```python
from build123d import *

# Parameters (mm, degrees)
F0_R     = 5
F1_DEPTH = 6.35
F0_R_2   = 11.43
F2_DEPTH = 3.175
F3_R     = 1.27


with BuildPart() as f1:
    # F0 (on Top) → F1 (new body)
    with BuildSketch(Plane.XY):
        Circle(F0_R)
    extrude(amount=F1_DEPTH)

    # F0 (on Top) → F2 (join)
    with BuildSketch(Plane.XY):
        Circle(F0_R_2)
        Circle(F0_R, mode=Mode.SUBTRACT)
    extrude(amount=F2_DEPTH)

    # F3
    f3_edges = [f1.edges().sort_by_distance(p)[0] for p in [
        (-11.43, 0, 0),
    ]]
    fillet(f3_edges, radius=F3_R)


solid = f1.part
```
Geometry: final body of the model. Coordinates: model frame, mm. A direction names the side the tool comes from. Round coordinates to 2 decimals unless told otherwise and drop trailing zeros. Write each loop counter-clockwise with the first axis right and the second up, starting at its lowest first coordinate (ties: lowest second). Pieces come first, ordered by that corner, then holes. Notation, with made-up numbers: (16, 17.25) -> (71, 17.25) arc R5 cw to (71, 21.25) -> close; hole circle Ø4 at (2.25, 71). An arc over 180 degrees is marked (long way). Return JSON: item names as keys, results as strings.
Q1. First-contact query: pin 1 Ø1.5 at (y, z) = (3.5, 2.5) entering from +X; pin 2 Ø1 at (x, z) = (3, 2.5) entering from +Y; pin 3 Ø1.5 at (x, y) = (5.5, -3.5) entering from +Z (3 decimals). Flat tips, straight axial feed; report the tip coordinate or a pass-through.
From the geometry:
{"pin 1": "x = 11.09", "pin 2": "y = 11.15", "pin 3": "z = 3.175"}
Q2. Section C-C on z = 4.25. Return the cut outline in (x, y).
From the geometry:
{"outline": "circle Ø10 at (0, 0)"}
Q3. Section A-A on y = 0. Return the cut outline in (x, z) (3 decimals).
From the geometry:
{"outline": "(-11.43, 1.27) arc R1.27 ccw to (-10.16, 0) -> (10.16, 0) arc R1.27 ccw to (11.43, 1.27) -> (11.43, 3.175) -> (5, 3.175) -> (5, 6.35) -> (-5, 6.35) -> (-5, 3.175) -> (-11.43, 3.175) -> close"}
Q4. Ray query, line 1 (Z direction, x = -9.25, y = -2.5) (3 decimals); line 2 (Y direction, x = -6.75, z = 3); line 3 (X direction, y = -1, z = 6.25). Return the intervals inside material, ascending.
From the geometry:
{"line 1": "0 to 3.175", "line 2": "-9.22 to 9.22", "line 3": "-4.9 to 4.9"}
Q5. Section D-D on z = 1. Return the cut outline in (x, y).
From the geometry:
{"outline": "circle Ø22.8 at (0, 0)"}
Q6. Set-up query: faces 1 (the cylindrical face through (10.902, 3.433, 2.209)), 2 (the flat face through (2, -5, 3.175)). Return all of +Z, -Z, +X, -X, +Y, -Y with unobstructed straight access to the full face (end or side cutting, diameter ignored); none if empty.
From the geometry:
{"face 1": "+Z, -Z", "face 2": "+Z"}
